from build123d import *

# Parameters (mm, degrees)
SKETCH_1_W          = 120
SKETCH_1_H          = 80
EXTRUDE_1_DEPTH     = 8
CUT_EXTRUDE_1_REACH = 10
SKETCH_2_R          = 5
EXTRUDE_2_DEPTH     = 200
CHAMFER_1_SIZE      = 30
CUT_EXTRUDE_3_REACH = 62
SKETCH_5_R          = 5
EXTRUDE_3_DEPTH     = 145
CHAMFER_2_SIZE      = 10
CUT_EXTRUDE_4_REACH = 57
SKETCH_7_R          = 1.75


with BuildPart() as part:
    # 草图1 → 凸台-拉伸1 (new body)
    with BuildSketch(Plane.XY):
        with Locations((60, 40)):
            Rectangle(SKETCH_1_W, SKETCH_1_H)
    extrude(amount=EXTRUDE_1_DEPTH)

    # 草图2 → 切除-拉伸1 (cut, up to next)
    with BuildSketch(Plane.XY.offset(8), mode=Mode.PRIVATE) as cut_extrude_1_sk1:
        with Locations((10, 65)):
            Circle(SKETCH_2_R)
    cut_extrude_1_tool1 = extrude(cut_extrude_1_sk1.sketch, amount=-CUT_EXTRUDE_1_REACH, mode=Mode.PRIVATE) & part.part
    add(cut_extrude_1_tool1.solids().sort_by_distance((10, 65, 8))[0], mode=Mode.SUBTRACT)
    # 草图2 → 切除-拉伸1 (cut, up to next)
    with BuildSketch(Plane.XY.offset(8), mode=Mode.PRIVATE) as cut_extrude_1_sk2:
        with Locations((10, 15)):
            Circle(SKETCH_2_R)
    cut_extrude_1_tool2 = extrude(cut_extrude_1_sk2.sketch, amount=-CUT_EXTRUDE_1_REACH, mode=Mode.PRIVATE) & part.part
    add(cut_extrude_1_tool2.solids().sort_by_distance((10, 15, 8))[0], mode=Mode.SUBTRACT)
    # 草图2 → 切除-拉伸1 (cut, up to next)
    with BuildSketch(Plane.XY.offset(8), mode=Mode.PRIVATE) as cut_extrude_1_sk3:
        with Locations((110, 15)):
            Circle(SKETCH_2_R)
    cut_extrude_1_tool3 = extrude(cut_extrude_1_sk3.sketch, amount=-CUT_EXTRUDE_1_REACH, mode=Mode.PRIVATE) & part.part
    add(cut_extrude_1_tool3.solids().sort_by_distance((110, 15, 8))[0], mode=Mode.SUBTRACT)
    # 草图2 → 切除-拉伸1 (cut, up to next)
    with BuildSketch(Plane.XY.offset(8), mode=Mode.PRIVATE) as cut_extrude_1_sk4:
        with Locations((110, 65)):
            Circle(SKETCH_2_R)
    cut_extrude_1_tool4 = extrude(cut_extrude_1_sk4.sketch, amount=-CUT_EXTRUDE_1_REACH, mode=Mode.PRIVATE) & part.part
    add(cut_extrude_1_tool4.solids().sort_by_distance((110, 65, 8))[0], mode=Mode.SUBTRACT)

    # 草图3 → 凸台-拉伸2 (add)
    with BuildSketch(Plane(origin=(0, 0, 0), x_dir=(-1, 0, 0), z_dir=(0, 0, -1))):
        with BuildLine():
            Line((-30, 20), (-82, 20))
            ThreePointArc((-82, 20), (-87.656854249, 22.343145751), (-90, 28))
            Line((-90, 28), (-90, 70))
            Line((-90, 70), (-86, 70))
            Line((-86, 70), (-86, 27.966747679))
            ThreePointArc((-86, 27.966747679), (-84.828427125, 25.138320554), (-82, 23.966747679))
            Line((-82, 23.966747679), (-30, 23.966747679))
            Line((-30, 23.966747679), (-30, 20))
        make_face()
    extrude(amount=EXTRUDE_2_DEPTH)

    # 倒角1
    chamfer_1_edges = [part.edges().sort_by_distance(p)[0] for p in [
        (30, 21.983373839, -200),
        (88, 70, -200),
    ]]
    chamfer(chamfer_1_edges, length=CHAMFER_1_SIZE)

    # 草图5 → 切除-拉伸3 (cut, up to next)
    with BuildSketch(Plane.XZ.offset(-20), mode=Mode.PRIVATE) as cut_extrude_3_sk1:
        with Locations((60, -70)):
            Circle(SKETCH_5_R)
    cut_extrude_3_tool1 = extrude(cut_extrude_3_sk1.sketch, amount=-CUT_EXTRUDE_3_REACH, mode=Mode.PRIVATE) & part.part
    add(cut_extrude_3_tool1.solids().sort_by_distance((60, 20, -70))[0], mode=Mode.SUBTRACT)
    # 草图5 → 切除-拉伸3 (cut, up to next)
    with BuildSketch(Plane.XZ.offset(-20), mode=Mode.PRIVATE) as cut_extrude_3_sk2:
        with Locations((60, -120)):
            Circle(SKETCH_5_R)
    cut_extrude_3_tool2 = extrude(cut_extrude_3_sk2.sketch, amount=-CUT_EXTRUDE_3_REACH, mode=Mode.PRIVATE) & part.part
    add(cut_extrude_3_tool2.solids().sort_by_distance((60, 20, -120))[0], mode=Mode.SUBTRACT)

    # 草图6 → 凸台-拉伸3 (add)
    with BuildSketch(Plane(origin=(90, 0, 0), x_dir=(0, 0, -1), z_dir=(1, 0, 0))):
        with BuildLine():
            Line((25, 47), (25, 28))
            Line((25, 28), (29, 28))
            Line((29, 28), (29, 47))
            ThreePointArc((29, 47), (30.171572875, 49.828427125), (33, 51))
            Line((33, 51), (85, 51))
            Line((85, 51), (85, 55))
            Line((85, 55), (33, 55))
            ThreePointArc((33, 55), (27.343145751, 52.656854249), (25, 47))
        make_face()
    extrude(amount=EXTRUDE_3_DEPTH)

    # 倒角2
    chamfer_2_edges = [part.edges().sort_by_distance(p)[0] for p in [
        (235, 53, -85),
        (235, 28, -27),
    ]]
    chamfer(chamfer_2_edges, length=CHAMFER_2_SIZE)

    # 草图7 → 切除-拉伸4 (cut, up to next)
    with BuildSketch(Plane(origin=(0, 55, 0), x_dir=(1, 0, 0), z_dir=(0, 1, 0)), mode=Mode.PRIVATE) as cut_extrude_4_sk1:
        with Locations((231, 65)):
            Circle(SKETCH_7_R)
    cut_extrude_4_tool1 = extrude(cut_extrude_4_sk1.sketch, amount=-CUT_EXTRUDE_4_REACH, mode=Mode.PRIVATE) & part.part
    add(cut_extrude_4_tool1.solids().sort_by_distance((231, 55, -65))[0], mode=Mode.SUBTRACT)
    # 草图7 → 切除-拉伸4 (cut, up to next)
    with BuildSketch(Plane(origin=(0, 55, 0), x_dir=(1, 0, 0), z_dir=(0, 1, 0)), mode=Mode.PRIVATE) as cut_extrude_4_sk2:
        with Locations((231, 44)):
            Circle(SKETCH_7_R)
    cut_extrude_4_tool2 = extrude(cut_extrude_4_sk2.sketch, amount=-CUT_EXTRUDE_4_REACH, mode=Mode.PRIVATE) & part.part
    add(cut_extrude_4_tool2.solids().sort_by_distance((231, 55, -44))[0], mode=Mode.SUBTRACT)
    # 草图7 → 切除-拉伸4 (cut, up to next)
    with BuildSketch(Plane(origin=(0, 55, 0), x_dir=(1, 0, 0), z_dir=(0, 1, 0)), mode=Mode.PRIVATE) as cut_extrude_4_sk3:
        with Locations((175, 44)):
            Circle(SKETCH_7_R)
    cut_extrude_4_tool3 = extrude(cut_extrude_4_sk3.sketch, amount=-CUT_EXTRUDE_4_REACH, mode=Mode.PRIVATE) & part.part
    add(cut_extrude_4_tool3.solids().sort_by_distance((175, 55, -44))[0], mode=Mode.SUBTRACT)
    # 草图7 → 切除-拉伸4 (cut, up to next)
    with BuildSketch(Plane(origin=(0, 55, 0), x_dir=(1, 0, 0), z_dir=(0, 1, 0)), mode=Mode.PRIVATE) as cut_extrude_4_sk4:
        with Locations((175, 65)):
            Circle(SKETCH_7_R)
    cut_extrude_4_tool4 = extrude(cut_extrude_4_sk4.sketch, amount=-CUT_EXTRUDE_4_REACH, mode=Mode.PRIVATE) & part.part
    add(cut_extrude_4_tool4.solids().sort_by_distance((175, 55, -65))[0], mode=Mode.SUBTRACT)


solid = part.part
Can you work these out from the model? Positions are in its coordinate system, mm. A direction names the side the tool comes from. Give positions to 0.01 mm unless a question says otherwise; leave off trailing zeros. Loops run counter-clockwise (first coordinate to the right, second up) from the corner with the lowest first, then second, coordinate; pieces in that order, holes last. Notation, with made-up numbers: (-4, -7) -> (36, -7) arc R20 cw to (36, 18) -> close; hole circle Ø5 at (59.5, -2.75). An arc over 180 degrees is marked (long way). Return JSON: item names as keys, results as strings.
Q1. I need wall thicknesses on probe 1 along Y at (x, z) = (10, 2); probe 2 along Z at (x, y) = (60, 22.35); probe 3 along X at (y, z) = (53.15, -65). Which ranges of each line are inside material? Lowest first, please.
Checks:
{"probe 1": "y = 0 to 10, 20 to 60, 70 to 80", "probe 2": "z = -200 to -125, -115 to -75, -65 to 8", "probe 3": "x = 86 to 173.25, 176.75 to 229.25, 232.75 to 235"}
Q2. We'd pull the mould along Z, two halves only. Please class faces 1 (the face through (230, 33, -27)), 2 (the face through (79, 23, -200)), 3 (the face through (161, 38, -25)): released by +Z, released by -Z, zero draft, split by the parting line, or undercut.
Checks:
{"face 1": "zero draft", "face 2": "released by -Z", "face 3": "undercut"}
Q3. I want a section at A-A, the plane y = 15. List the corners of the cut face in (x, z) for me, then the cut area to 3 significant figures.
Checks:
{"outline": "(0, 0) -> (5, 0) -> (5, 8) -> (0, 8) -> close; (15, 0) -> (105, 0) -> (105, 8) -> (15, 8) -> close; (115, 0) -> (120, 0) -> (120, 8) -> (115, 8) -> close", "area": "800 mm2"}
Q4. I want a section at D-D, the plane z = -166. List the corners of the cut face in (x, y) for me.
Checks:
{"outline": "(30, 20) -> (82, 20) arc R8 ccw to (90, 28) -> (90, 70) -> (86, 70) -> (86, 27.97) arc R4 cw to (82, 23.97) -> (30, 23.97) -> close"}
Q5. On a 3-axis mill with a long thin cutter (end or side, diameter ignored), from which of +Z, -Z, +X, -X, +Y, -Y can I reach the whole of each face in a straight line? I mean faces 4 (the face through (56, 23.967, -99)), 5 (the face through (161.485, 52.719, -27.406)), 6 (the face through (120, 39, 4)). Say none if no direction works.
Checks:
{"face 4": "-Z, -X, +Y", "face 5": "+X, +Y", "face 6": "+Z, +X, +Y, -Y"}
Q6. I want a section at C-C, the plane x = 10. List the corners of the cut face in (y, z) for me.
Checks:
{"outline": "(0, 0) -> (10, 0) -> (10, 8) -> (0, 8) -> close; (20, 0) -> (60, 0) -> (60, 8) -> (20, 8) -> close; (70, 0) -> (80, 0) -> (80, 8) -> (70, 8) -> close"}
Q7. I want a section at B-B, the plane x = 110. List the corners of the cut face in (y, z) for me, then the cut area to 3 significant figures.
Checks:
{"outline": "(0, 0) -> (10, 0) -> (10, 8) -> (0, 8) -> close; (20, 0) -> (60, 0) -> (60, 8) -> (20, 8) -> close; (28, -29) -> (47, -29) arc R4 cw to (51, -33) -> (51, -85) -> (55, -85) -> (55, -33) arc R8 ccw to (47, -25) -> (28, -25) -> close; (70, 0) -> (80, 0) -> (80, 8) -> (70, 8) -> close", "area": "802 mm2"}
Q8. For pin 1 Ø12 at (y, z) = (41.5, -129.5) entering from +X; pin 2 Ø21 at (x, y) = (195, 38.5) entering from -Z; pin 3 Ø3 at (y, z) = (25, -120) entering from +X, each with a flat end and sliding along its axis, tell me the tip position at first contact or that it passes through.
Checks:
{"pin 1": "stops at x = 90", "pin 2": "stops at z = -29.54", "pin 3": "stops at x = 89.86"}
